Input: part model. Units: mm. Frame: model coordinates. A direction names the side the tool comes from. Coordinates: 2 decimals unless noted, no trailing zeros. Loops run counter-clockwise (first coordinate to the right, second up) from the corner with the lowest first, then second, coordinate; pieces in that order, holes last. Notation, with made-up numbers: M -9.75,78.25 L 12.25,78.25 A30 cw 12.25,108.25 Z; hole C -12,-7.5 d5. An arc over 180 degrees is marked long. Use a Markdown table: item, result. Add a question column.
1. Draft query along X for faces 1 (the flat face through (-15.357, 9.437, -19.517)), 2 (the flat face through (-58, 14, 0)), 3 (the flat face through (-55, 8, -25)). Return one class per face: +X half, -X half, draft (parallel to the pull), parting line (faces both ways), or undercut.
2. Section D-D on x = 0. Output: boundary loops of the cut face in (y, z).
3. Section A-A on z = 5.5. State how many separate pieces and enclosed holes the cut face has, then the cut area to 3 significant figures.
4. Set-up query: faces 4 (the flat face through (-46, 10.7, 9)), 5 (the flat face through (-63.43, 4.49, 26.23)), 6 (the flat face through (-0.4, 8.5, -26)). Return all of +Z, -Z, +X, -X, +Y, -Y with unobstructed straight access to the full face (end or side cutting, diameter ignored); none if empty.
5. Pin query (flat end, axial travel): pin 1 (6 mm diameter, centred on x = -20, z = 16, fed in from +Y); pin 2 (3 mm diameter, centred on y = 8.5, z = 25, fed in from +X); pin 3 (1 mm diameter, centred on y = 7, z = -24.5, fed in from +X); pin 4 (4 mm diameter, centred on x = -52, z = -25, fed in from +Y). Return the tip coordinate at first contact, or that it passes through.
6. Line query: L1, parallel to X at y = 4.5, z = -15.5; L2, parallel to Z at x = -22, y = 7.75; L3, parallel to Z at x = -51, y = 2.5. Output: solid intervals per line, ascending. Write a range as [from, to].
7. Section B-B on x = -35. Output: boundary loops of the cut face in (y, z).
```python
from build123d import *

# Parameters (mm, degrees)
SKETCH1_R                = 11.5
SKETCH1_R_2              = 1.6
BOSS_EXTRUDE1_DEPTH      = 5
BOSS_EXTRUDE2_DEPTH      = 9
SKETCH3_R                = 20.8
SKETCH3_R_2              = 12.1
CUT_EXTRUDE1_DEPTH       = 3.3
SKETCH4_R                = 6.85
CUT_EXTRUDE2_DEPTH       = 4
SKETCH5_R                = 7.85
CUT_EXTRUDE3_DEPTH       = 10
CUT_EXTRUDE4_DEPTH       = 10
SKETCH7_R                = 2.15
CUT_EXTRUDE5_DEPTH       = 79.90393653
CHAMFER1_SIZE            = 10
CHAMFER2_SIZE            = 14.66
CHAMFER3_SIZE            = 5
SKETCH8_R                = 3
CUT_EXTRUDE6_DEPTH       = 1.5
BOSS_EXTRUDE3_DEPTH      = 22
BOSS_EXTRUDE3_DEPTH_BACK = 1.5
BOSS_EXTRUDE4_DEPTH      = 13.73
SKETCH12_R               = 1
CUT_EXTRUDE7_DEPTH       = 13.73
SKETCH13_R               = 2.5
CUT_EXTRUDE8_DEPTH       = 1.5
FILLET1_R                = 1


# Some blends are built 0.0001 mm under size
with BuildPart() as part:
    # Sketch1 → Boss-Extrude1 (new body)
    with BuildSketch(Plane(origin=(0, 0, 0), x_dir=(1, 0, 0), z_dir=(0, 1, 0))):
        Polygon((24.5, 22.5), (24.5, -22.5), (-10.19, -22.5), (-10.19, -33.66), (-70.66, -33.66), (-70.66, 33.66), (6.9, 33.66), (6.9, 22.5), align=None)
        with Locations(Location((0, 0, 0), (0, 0, 270))):
            Circle(SKETCH1_R, mode=Mode.SUBTRACT)
        with Locations(Location((15.5, 15.5, 0), (0, 0, 270))):
            Circle(SKETCH1_R_2, mode=Mode.SUBTRACT)
        with Locations(Location((15.5, -15.5, 0), (0, 0, 270))):
            Circle(SKETCH1_R_2, mode=Mode.SUBTRACT)
        with Locations(Location((-15.5, -15.5, 0), (0, 0, 270))):
            Circle(SKETCH1_R_2, mode=Mode.SUBTRACT)
        with Locations(Location((-15.5, 15.5, 0), (0, 0, 270))):
            Circle(SKETCH1_R_2, mode=Mode.SUBTRACT)
    extrude(amount=BOSS_EXTRUDE1_DEPTH)

    # Sketch2 → Boss-Extrude2 (add)
    with BuildSketch(Plane(origin=(0, 5, 0), x_dir=(1, 0, 0), z_dir=(0, 1, 0))):
        with BuildLine():
            Line((-10.19, -33.66), (-10.19, -22.5))
            Line((-10.19, -22.5), (-20.381763801, -16.615782426))
            ThreePointArc((-20.381763801, -16.615782426), (-45.992259152, -21.711500992), (-60.5, 0))
            Line((-60.5, 0), (-70.66, 0))
            Line((-70.66, 0), (-70.66, -33.66))
            Line((-70.66, -33.66), (-10.19, -33.66))
        make_face()
        with BuildLine():
            ThreePointArc((-60.5, 0), (-45.992259152, -21.711500992), (-20.381763801, -16.615782426))
            ThreePointArc((-20.381763801, -16.615782426), (-15.288499008, -8.992259152), (-13.5, 0))
            Line((-13.5, 0), (-60.5, 0))
        make_face()
        with BuildLine():
            Line((-60.5, 0), (-13.5, 0))
            ThreePointArc((-13.5, 0), (-15.288499008, 8.992259152), (-20.381763801, 16.615782426))
            ThreePointArc((-20.381763801, 16.615782426), (-45.992259152, 21.711500992), (-60.5, 0))
        make_face()
        with BuildLine():
            Line((-70.66, 0), (-60.5, 0))
            ThreePointArc((-60.5, 0), (-45.992259152, 21.711500992), (-20.381763801, 16.615782426))
            Line((-20.381763801, 16.615782426), (-10.19, 22.5))
            Line((-10.19, 22.5), (-16.633229004, 33.66))
            Line((-16.633229004, 33.66), (-70.66, 33.66))
            Line((-70.66, 33.66), (-70.66, 0))
        make_face()
    extrude(amount=BOSS_EXTRUDE2_DEPTH)

    # Sketch3 → Cut-Extrude1 (cut)
    with BuildSketch(Plane(origin=(0, 14, 0), x_dir=(1, 0, 0), z_dir=(0, 1, 0))):
        with Locations(Location((-37, 0, 0), (0, 0, 270))):
            Circle(SKETCH3_R)
        with Locations(Location((-37, 0, 0), (0, 0, 270))):
            Circle(SKETCH3_R_2, mode=Mode.SUBTRACT)
    extrude(amount=-CUT_EXTRUDE1_DEPTH, mode=Mode.SUBTRACT)

    # Sketch4 → Cut-Extrude2 (cut)
    with BuildSketch(Plane(origin=(0, 14, 0), x_dir=(1, 0, 0), z_dir=(0, 1, 0))):
        with Locations(Location((-37, 0, 0), (0, 0, 270))):
            Circle(SKETCH4_R)
    extrude(amount=-CUT_EXTRUDE2_DEPTH, mode=Mode.SUBTRACT)

    # Sketch5 → Cut-Extrude3 (cut)
    with BuildSketch(Plane.XZ):
        with Locations(Location((-37, 0, 0), (0, 0, 270))):
            Circle(SKETCH5_R)
    extrude(amount=-CUT_EXTRUDE3_DEPTH, mode=Mode.SUBTRACT)

    # Sketch6 → Cut-Extrude4 (cut)
    with BuildSketch(Plane(origin=(0, 14, 0), x_dir=(1, 0, 0), z_dir=(0, 1, 0))):
        Polygon((-55, 26.732050808), (-52, 28.464101615), (-49, 26.732050808), (-49, 23.267949192), (-52, 21.535898385), (-55, 23.267949192), align=None)
        Polygon((-22, 28.464101615), (-25, 26.732050808), (-25, 23.267949192), (-22, 21.535898385), (-19, 23.267949192), (-19, 26.732050808), align=None)
        Polygon((-52, -21.535898385), (-55, -23.267949192), (-55, -26.732050808), (-52, -28.464101615), (-49, -26.732050808), (-49, -23.267949192), align=None)
        Polygon((-19, -26.732050808), (-22, -28.464101615), (-25, -26.732050808), (-25, -23.267949192), (-22, -21.535898385), (-19, -23.267949192), align=None)
        Polygon((-65, -13.267949192), (-62, -11.535898385), (-59, -13.267949192), (-59, -16.732050808), (-62, -18.464101615), (-65, -16.732050808), align=None)
        Polygon((-62, 11.535898385), (-59, 13.267949192), (-59, 16.732050808), (-62, 18.464101615), (-65, 16.732050808), (-65, 13.267949192), align=None)
    extrude(amount=-CUT_EXTRUDE4_DEPTH, mode=Mode.SUBTRACT)

    # Sketch7 → Cut-Extrude5 (cut, through all)
    with BuildSketch(Plane(origin=(0, 4, 0), x_dir=(1, 0, 0), z_dir=(0, 1, 0))):
        with Locations(Location((-62, -15, 0), (0, 0, 270))):
            Circle(SKETCH7_R)
        with Locations(Location((-52, -25, 0), (0, 0, 270))):
            Circle(SKETCH7_R)
        with Locations(Location((-22, -25, 0), (0, 0, 270))):
            Circle(SKETCH7_R)
        with Locations(Location((-62, 15, 0), (0, 0, 270))):
            Circle(SKETCH7_R)
        with Locations(Location((-52, 25, 0), (0, 0, 270))):
            Circle(SKETCH7_R)
        with Locations(Location((-22, 25, 0), (0, 0, 270))):
            Circle(SKETCH7_R)
    extrude(amount=-CUT_EXTRUDE5_DEPTH, mode=Mode.SUBTRACT)

    # Chamfer1
    # the kernel refuses this chamfer: 10 mm, written as the material it takes off along each edge
    with BuildSketch(Plane(origin=(-10.19, 39.71682988, 33.66), x_dir=(0.027495876610586317, 0, -0.9996219169112968), z_dir=(0, -1, 0))) as chamfer1_piece_1:
        Polygon((CHAMFER1_SIZE * 0.999621916911, -CHAMFER1_SIZE * 0.0274958766106), (-CHAMFER1_SIZE * 0.0274958766106, -CHAMFER1_SIZE * 0.999621916911), (0, 0), align=None)
    extrude(amount=65.433659759, mode=Mode.SUBTRACT)
    with BuildSketch(Plane(origin=(9.083600876, 14, -33.66), x_dir=(0, -0.9996219169112968, -0.027495876610586317), z_dir=(-1, 0, 0))) as chamfer1_piece_2:
        Polygon((CHAMFER1_SIZE * 0.999621916911, CHAMFER1_SIZE * 0.0274958766106), (-CHAMFER1_SIZE * 0.0274958766106, CHAMFER1_SIZE * 0.999621916911), (0, 0), align=None)
    extrude(amount=105.460430755, mode=Mode.SUBTRACT)
    with BuildSketch(Plane(origin=(-96.37682988, 14, 33.66), x_dir=(0, -0.9996219169112968, 0.027495876610586317), z_dir=(1, 0, 0))) as chamfer1_piece_3:
        Polygon((CHAMFER1_SIZE * 0.999621916911, CHAMFER1_SIZE * 0.0274958766106), (-CHAMFER1_SIZE * 0.0274958766106, CHAMFER1_SIZE * 0.999621916911), (0, 0), align=None)
    extrude(amount=111.903659759, mode=Mode.SUBTRACT)
    with BuildSketch(Plane(origin=(-70.66, 14, -59.37682988), x_dir=(-0.027495876610586317, -0.9996219169112968, 0), z_dir=(0, 0, 1))) as chamfer1_piece_4:
        Polygon((CHAMFER1_SIZE * 0.999621916911, CHAMFER1_SIZE * 0.0274958766106), (-CHAMFER1_SIZE * 0.0274958766106, CHAMFER1_SIZE * 0.999621916911), (0, 0), align=None)
    extrude(amount=118.753659759, mode=Mode.SUBTRACT)

    # Chamfer2
    chamfer2_edges = [part.edges().sort_by_distance(p)[0] for p in [
        (-70.66, 2, 33.66),
        (-70.66, 2, -33.66),
    ]]
    chamfer(chamfer2_edges, length=CHAMFER2_SIZE)

    # Chamfer3
    chamfer3_edges = [part.edges().sort_by_distance(p)[0] for p in [
        (24.5, 5, 0),
    ]]
    chamfer(chamfer3_edges, length=CHAMFER3_SIZE - 0.0001)  # a hair under: the kernel refuses the full size

    # Sketch8 → Cut-Extrude6 (cut)
    with BuildSketch(Plane(origin=(0, 5, 0), x_dir=(1, 0, 0), z_dir=(0, 1, 0))):
        with Locations(Location((15.5, 15.5, 0), (0, 0, 270))):
            Circle(SKETCH8_R)
        with Locations(Location((-15.5, 15.5, 0), (0, 0, 270))):
            Circle(SKETCH8_R)
        with Locations(Location((-15.5, -15.5, 0), (0, 0, 270))):
            Circle(SKETCH8_R)
        with Locations(Location((15.5, -15.5, 0), (0, 0, 270))):
            Circle(SKETCH8_R)
    extrude(amount=-CUT_EXTRUDE6_DEPTH, mode=Mode.SUBTRACT)

    # Sketch9 → Boss-Extrude3 (add, two sides: drawn at the far end of the back side and taken through both)
    with BuildSketch(Plane(origin=(0, 5, 0), x_dir=(1, 0, 0), z_dir=(0, 1, 0)).offset(-BOSS_EXTRUDE3_DEPTH_BACK)):
        Polygon((6.9, 33.66), (6.9, 29.56), (-6.8, 29.56), (-7.995869238, 30.755869238), (-6.8, 33.66), align=None)
    extrude(amount=BOSS_EXTRUDE3_DEPTH + BOSS_EXTRUDE3_DEPTH_BACK)

    # Sketch10 → Boss-Extrude4 (add)
    with BuildSketch(Plane(origin=(6.9, 0, 0), x_dir=(0, 0, -1), z_dir=(1, 0, 0))):
        Polygon((22.5, 5), (29.56, 12.06), (29.56, 5), align=None)
    extrude(amount=-BOSS_EXTRUDE4_DEPTH)

    # Sketch12 → Cut-Extrude7 (cut)
    with BuildSketch(Plane.XY.offset(-29.56)):
        with Locations((-4, 21.35)):
            Circle(SKETCH12_R)
        with Locations((-4, 14.85)):
            Circle(SKETCH12_R)
    extrude(amount=-CUT_EXTRUDE7_DEPTH, mode=Mode.SUBTRACT)

    # Sketch13 → Cut-Extrude8 (cut)
    with BuildSketch(Plane(origin=(0, 0, -33.66), x_dir=(-1, 0, 0), z_dir=(0, 0, -1))):
        with Locations((4, 14.85)):
            Circle(SKETCH13_R)
        with Locations((4, 21.35)):
            Circle(SKETCH13_R)
    extrude(amount=-CUT_EXTRUDE8_DEPTH, mode=Mode.SUBTRACT)

    # Fillet1
    fillet1_edges = [part.edges().sort_by_distance(p)[0] for p in [
        (6.9, 13.5, -33.66),
        (6.9, 19.53, -29.56),
        (6.9, 8.53, -26.03),
    ]]
    fillet(fillet1_edges, radius=FILLET1_R)


solid = part.part
```
Answers below:
| question | item | result |
|---|---|---|
| 1 | face 1 | +X half |
| 1 | face 2 | draft |
| 1 | face 3 | undercut |
| 2 | outline | M 0,-33.66 L 27,-33.66 L 27,-29.56 L 12.06,-29.56 L 5,-22.5 L 5,-11.5 L 0,-11.5 Z; M 0,11.5 L 5,11.5 L 5,22.5 L 0,22.5 Z |
| 3 | separate pieces | 3 |
| 3 | enclosed holes | 0 |
| 3 | area | 615 mm² |
| 4 | face 4 | +Y |
| 4 | face 5 | +Z, -X, +Y, -Y |
| 4 | face 6 | +Z, +X, +Y |
| 5 | pin 1 | stops at y = 14 |
| 5 | pin 2 | stops at x = -10.19 |
| 5 | pin 3 | stops at x = 6.77 |
| 5 | pin 4 | passes through |
| 6 | L1 | x = [-70.16, -65], [-59, -18.5], [-12.5, 12.5], [18.5, 20] |
| 6 | L2 | z = [-29.91, -28.46], [-21.54, 21.54], [28.46, 29.91] |
| 6 | L3 | z = [-33.66, -26.9], [-23.1, 23.1], [26.9, 33.66] |
| 7 | outline | M 0,-33.66 L 4,-33.66 L 14,-23.66 L 14,-20.7 L 10.7,-20.7 L 10.7,-11.93 L 14,-11.93 L 14,-6.55 L 10,-6.55 L 10,-7.59 L 0,-7.59 Z; M 0,7.59 L 10,7.59 L 10,6.55 L 14,6.55 L 14,11.93 L 10.7,11.93 L 10.7,20.7 L 14,20.7 L 14,23.66 L 4,33.66 L 0,33.66 Z |
